Here's how the part is built. I have some questions about the finished solid (model axes, mm). A direction names the side the tool comes from. Give positions to 0.01 mm unless a question says otherwise; leave off trailing zeros. Loops run counter-clockwise (first coordinate to the right, second up) from the corner with the lowest first, then second, coordinate; pieces in that order, holes last. Notation, with made-up numbers: (78.5, -5) - (126.5, -5) arc R24 ccw to (126.5, 13) - close; hole circle Ø4 at (20.25, 28). An arc over 180 degrees is marked (long way). Use one line per item in the form item = value.
Autodesk Inventor part; units mm, degrees
ref_plane "YZ Plane" through (0, 0, 0) normal (1, 0, 0) x (0, 1, 0)
ref_plane "XZ Plane" through (0, 0, 0) normal (0, 1, 0) x (-1, 0, 0)
ref_plane "XY Plane" through (0, 0, 0) normal (0, 0, 1) x (1, 0, 0)
sketch "Sketch1" plane through (0, 0, 0) normal (0, 0, 1) x (1, 0, 0)
  line L0 (2.794, -1.6131) -> (0, -3.2262)
  line L1 (0, -3.2262) -> (-2.794, -1.6131)
  line L2 (-2.794, -1.6131) -> (-2.794, 1.6131)
  line L3 (-2.794, 1.6131) -> (0, 3.2262)
  line L4 (0, 3.2262) -> (2.794, 1.6131)
  line L5 (2.794, 1.6131) -> (2.794, -1.6131)
  point P0 (0, 0)
  point P1 (0, 0)
  point P2 (2.794, 0)
  dimension "d0" = 5.588
extrude "Extrusion1" add sketch "Sketch1" along normal mid plane 25.4
sketch "Sketch2" plane through (2.794, -1.6131, 12.7) normal (1, 0, 0) x (0, 0, -1)
  line L0 (0, 0) -> (0, 3.2262) construction
  circle A0 centre (3.0551, 1.6131) radius 1.016
  point P0 (12.7, 1.6131)
  dimension "d3" = 2.032
  dimension "d4" = 3.0551
extrude "Extrusion2" cut sketch "Sketch2" against normal through all
sketch "Sketch3" plane through (0, 0, -12.7) normal (0, 0, -1) x (-1, 0, 0)
  circle A0 centre (0, 0) radius 1.397
  dimension "d9" = 2.794
extrude "Extrusion3" cut sketch "Sketch3" against normal blind 19.05
properties part number "tensioners"
(1) If we section it at C-C (x = 1.15): List the corners of the cut face in (y, z) for me.
Geometry says:
outline = (-2.56, -12.7) - (-0.79, -12.7) - (-0.79, 6.35) - (0.79, 6.35) - (0.79, -12.7) - (2.56, -12.7) - (2.56, 12.7) - (-2.56, 12.7) - close; hole circle Ø2.03 at (0, 9.64)
(2) For P1, Ø2, axis at x = 0, y = 0, coming from the -Z side; P2, Ø2.5, axis at y = 0, z = 9.64, coming from the -X side; P3, Ø2, axis at x = 0.5, z = -9, coming from the -Y side, each with a flat end and sliding along its axis, tell me the tip position at first contact or that it passes through.
Geometry says:
P1 = 6.35
P2 = -2.79
P3 = -3.23
(3) Thinking about a two-plate mould opening in X: for faces 3 (the flat face through (-2.794, 0, 0)), 4 (the cylindrical face through (1.11, -0.85, -3.31)), 5 (the flat face through (2.794, 0, 0)), which applies, pulls with the +X half, pulls with the -X half, needs draft (parallel to the pull), parting line crosses it, or undercut?
Geometry says:
face_3 = pulls with the -X half
face_4 = undercut
face_5 = pulls with the +X half
(4) If I drill on probe 1 along Y at (x, z) = (-0.6, -0.5); probe 2 along X at (y, z) = (1, -10); probe 3 along X at (y, z) = (-0.25, 6), over which ranges is the centre line in solid material (lowest first)?
Geometry says:
probe_1 = -2.88 to -1.26, 1.26 to 2.88
probe_2 = -2.79 to -0.98, 0.98 to 2.79
probe_3 = -2.79 to -1.37, 1.37 to 2.79
(5) If we section it at B-B (z = -5.5): List the corners of the cut face in (x, y) for me.
Geometry says:
outline = (-2.79, -1.61) - (0, -3.23) - (2.79, -1.61) - (2.79, 1.61) - (0, 3.23) - (-2.79, 1.61) - close; hole circle Ø2.79 at (0, 0)
(6) If we section it at A-A (y = 0): List the corners of the cut face in (x, z) for me, plus the area to 3 significant figures.
Geometry says:
outline = (-2.79, -12.7) - (-1.4, -12.7) - (-1.4, 6.35) - (1.4, 6.35) - (1.4, -12.7) - (2.79, -12.7) - (2.79, 8.63) - (-2.79, 8.63) - close; (-2.79, 10.66) - (2.79, 10.66) - (2.79, 12.7) - (-2.79, 12.7) - close
area = 77.4 mm²
(7) If we section it at D-D (x = 2.2): List the corners of the cut face in (y, z) for me, plus the area to 3 significant figures.
Geometry says:
outline = (-1.96, -12.7) - (1.96, -12.7) - (1.96, 12.7) - (-1.96, 12.7) - close; hole circle Ø2.03 at (0, 9.64)
area = 96.1 mm²
(8) For faces 1 (the flat face through (-1.38, -2.43, -0.18)), 2 (the flat face through (0, 0, 6.35)), which set-ups out of +Z, -Z, +X, -X, +Y, -Y let a thin tool reach every point of the face, with its end or its side?
Geometry says:
face_1 = +Z, -Z, -X, -Y
face_2 = -Z
